from build123d import *

# Parameters (mm, degrees)
BOX001_W             = 0.6
BOX001_H             = 0.6
BOX001_DEPTH         = 5
BOX002_W             = 0.6
BOX002_H             = 0.6
BOX002_DEPTH         = 5
CYLINDER004_R        = 2.5
CYLINDER004_DEPTH    = 6.1
BOX_W                = 10
BOX_H                = 10
BOX_DEPTH            = 10
CYLINDER005_R        = 2.9
CYLINDER005_DEPTH    = 1
FUSION002_ROLL_ANGLE = -90


with BuildPart() as led_pin1:
    # Box001 → Box001 (new body)
    with BuildSketch(Plane(origin=(-0.3, 1.27, -5), x_dir=(1, 0, 0), z_dir=(0, 0, 1))):
        with Locations((0.3, 0.3)):
            Rectangle(BOX001_W, BOX001_H)
    extrude(amount=BOX001_DEPTH)


with BuildPart() as led_pin2:
    # Box002 → Box002 (new body)
    with BuildSketch(Plane(origin=(-0.3, -1.27, -5), x_dir=(1, 0, 0), z_dir=(0, 0, 1))):
        with Locations((0.3, 0.3)):
            Rectangle(BOX002_W, BOX002_H)
    extrude(amount=BOX002_DEPTH)


with BuildPart() as led_cyl:
    # Cylinder004 → Cylinder004 (new body)
    with BuildSketch(Plane.XY):
        Circle(CYLINDER004_R)
    extrude(amount=CYLINDER004_DEPTH)


with BuildPart() as led_key_cut:
    # Box → Box (new body)
    with BuildSketch(Plane(origin=(-5, 2.5, 0), x_dir=(1, 0, 0), z_dir=(0, 0, 1))):
        with Locations((5, 5)):
            Rectangle(BOX_W, BOX_H)
    extrude(amount=BOX_DEPTH)


with BuildPart() as cut001:
    # Cylinder005 → Cylinder005 (new body)
    with BuildSketch(Plane.XY):
        Circle(CYLINDER005_R)
    extrude(amount=CYLINDER005_DEPTH)

    # Cut001: cut led-key-cut
    add(led_key_cut.part, mode=Mode.SUBTRACT)


with BuildPart() as led5mm:
    # Sphere → Sphere (revolve)
    with BuildSketch(Plane(origin=(0, 0, 6.1), x_dir=(1, 0, 0), z_dir=(0, -1, 0))):
        with BuildLine():
            ThreePointArc((0, -2.5), (2.5, 0), (0, 2.5))
            Line((0, 2.5), (0, -2.5))
        make_face()
    revolve(axis=Axis((0, 0, 6.1), (0, 0, 1)))

    # Fusion001: union led-cyl, Cut001
    add(led_cyl.part)
    add(cut001.part)

    # Fusion002: union led-pin1, led-pin2
    add(led_pin1.part)
    add(led_pin2.part)


with BuildPart() as led5mm_1:
    # Fusion002 roll: moved
    add(led5mm.part.rotate(Axis((0, 0, 0), (1, 0, 0)), FUSION002_ROLL_ANGLE))


with BuildPart() as led5mm_2:
    # Fusion002 placement: moved
    add(led5mm_1.part.moved(Location((33.37, 6.8, 6.38))))


solid = led5mm_2.part
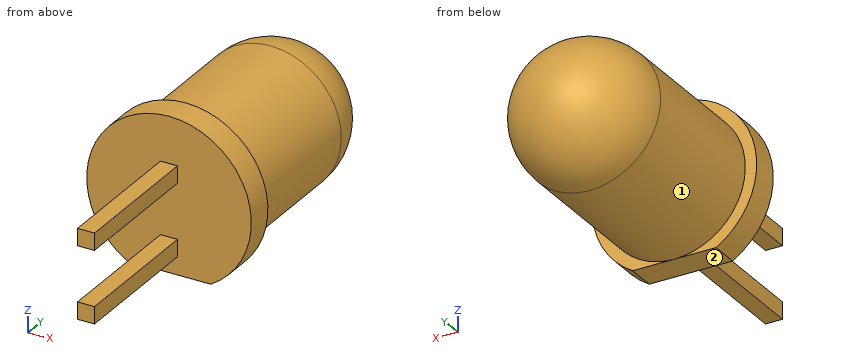
Here's how the part is built. I have some questions about the finished solid (model axes, mm). Face numbers are marked on the shaded views. A direction names the side the tool comes from. Coordinates: 2 decimals unless noted, no trailing zeros. Write each loop counter-clockwise with the first axis right and the second up, starting at its lowest first coordinate (ties: lowest second). Pieces come first, ordered by that corner, then holes.
Item 1: On a 3-axis mill with a long thin cutter (end or side, diameter ignored), from which of +Z, -Z, +X, -X, +Y, -Y can I reach the whole of each face in a straight line? I mean the marked faces 1 and 2. Say none if no direction works.
Item 2: I want a section at B-B on z = 6.38. Write out the boundary of the cut face in (x, y), and give its area (3 significant figures).
Item 3: If I drill on line 1 (Z direction, x = 33.4, y = 5.5); line 2 (X direction, y = 6.75, z = 4.65); line 3 (Y direction, x = 32.85, z = 9), over which ranges is the centre line in solid material (lowest first)?
Item 4: I want a section at D-D on y = 7. Write out the boundary of the cut face in (x, z).
Item 5: I want a section at A-A on y = 3. Write out the boundary of the cut face in (x, z).
Item 6: I want a section at C-C on x = 32.75. Write out the boundary of the cut face in (y, z).
Item 7: Will these pins go through, and if not, where does the flat tip stop? pin 1 (0.5 mm diameter, centred on y = 4, z = 5, fed in from -X); pin 2 (3 mm diameter, centred on x = 35.5, z = 5.5, fed in from +Y); pin 3 (3 mm diameter, centred on y = 9, z = 8, fed in from -X); pin 4 (1 mm diameter, centred on y = 5.5, z = 8.5, fed in from +X).
Findings below:
1. face 1: +Y
1. face 2: -Z, +X, -X, +Y, -Y
2. outline: (30.47, 6.8) - (36.27, 6.8) - (36.27, 7.8) - (35.87, 7.8) - (35.87, 12.9) arc R2.5 ccw to (30.87, 12.9) - (30.87, 7.8) - (30.47, 7.8) - close
2. area: 41.1 mm2
3. line 1: z = 4.51 to 5.11, 7.05 to 7.65
3. line 2: x = 33.07 to 33.67
3. line 3: y = 6.8 to 7.8
4. outline: (31.9, 3.88) - (34.84, 3.88) arc R2.9 ccw (long way) to start
5. outline: (33.07, 4.51) - (33.67, 4.51) - (33.67, 5.11) - (33.07, 5.11) - close; (33.07, 7.05) - (33.67, 7.05) - (33.67, 7.65) - (33.07, 7.65) - close
6. outline: (6.8, 3.88) - (7.8, 3.88) - (7.8, 3.96) - (12.9, 3.96) arc R2.42 ccw to (12.9, 8.8) - (7.8, 8.8) - (7.8, 9.21) - (6.8, 9.21) - close
7. pin 1: stops at x = 33.07
7. pin 2: stops at y = 15.27
7. pin 3: stops at x = 30.56
7. pin 4: passes through
